from build123d import *

# Parameters (mm, degrees)
F1_DEPTH = 10
F2_R     = 10
F3_R     = 10


with BuildPart() as f1:
    # F0 (on Top) → F1 (new body)
    with BuildSketch(Plane.XY):
        with BuildLine():
            Line((-14.6, -8.429314), (-14.6, -20.293841))
            ThreePointArc((-14.6, -20.293841), (0, -25), (14.6, -20.293841))
            Line((14.6, -20.293841), (14.6, -8.429314))
            Line((14.6, -8.429314), (0, -16.858628))
            Line((0, -16.858628), (-14.6, -8.429314))
        make_face()
        with BuildLine():
            ThreePointArc((14.6, -20.293841), (22.248595, -11.401754), (25, 0))
            ThreePointArc((25, 0), (-11.401754, 22.248595), (-14.6, -20.293841))
            Line((-14.6, -20.293841), (-14.6, -8.429314))
            Line((-14.6, -8.429314), (-14.6, 8.429314))
            Line((-14.6, 8.429314), (0, 16.858628))
            Line((0, 16.858628), (14.6, 8.429314))
            Line((14.6, 8.429314), (14.6, -8.429314))
            Line((14.6, -8.429314), (14.6, -20.293841))
        make_face()
        with BuildLine():
            ThreePointArc((14.6, -20.293841), (0, -25), (-14.6, -20.293841))
            Line((-14.6, -20.293841), (-14.6, -104.361953))
            Line((-14.6, -104.361953), (14.6, -104.361953))
            Line((14.6, -104.361953), (14.6, -20.293841))
        make_face()
    extrude(amount=F1_DEPTH)

    # F2
    f2_edges = [f1.edges().sort_by_distance(p)[0] for p in [
        (14.6, -20.293841, 5),
    ]]
    fillet(f2_edges, radius=F2_R)

    # F3
    f3_edges = [f1.edges().sort_by_distance(p)[0] for p in [
        (-14.6, -20.293841, 5),
        (-14.6, -104.361953, 5),
        (14.6, -104.361953, 5),
    ]]
    fillet(f3_edges, radius=F3_R)


solid = f1.part
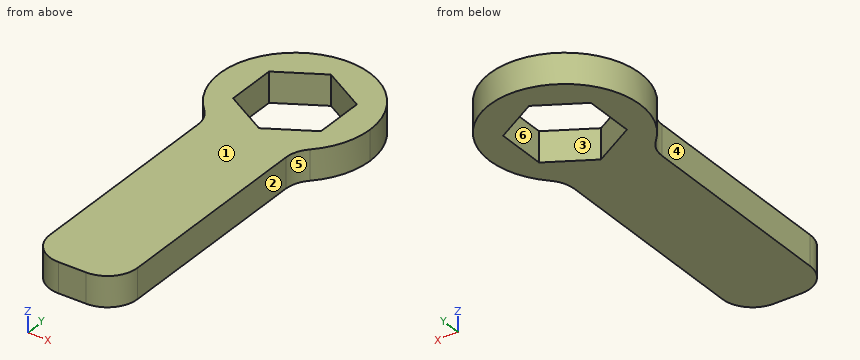
Input: part model. Units: mm. Frame: model coordinates. Face numbers are marked on the shaded views. A direction names the side the tool comes from. Give positions to 0.01 mm unless a question says otherwise; leave off trailing zeros. Order: outer loops, then holes, each group sorted by start corner. A loop starts at its lowest first (then second) coordinate and runs counter-clockwise, first axis right, second up. Notation, with made-up numbers: (67.5, 82.25) -> (89.5, 82.25) arc R27 ccw to (89.5, 109.25) -> close; hole circle Ø3 at (-10, 50.5). An arc over 180 degrees is marked (long way). Use one line per item in the form item = value.
1) Mould query, pull axis X, two halves, no side actions, for the marked faces 1, 2, 3 and 4. Classes: pulls with the +X half, pulls with the -X half, needs draft (parallel to the pull), parting line crosses it, or undercut.
Response values:
face_1 = needs draft
face_2 = pulls with the +X half
face_3 = undercut
face_4 = pulls with the -X half
2) Section C-C, the plane x = 1.5. Return loops of the section in (y, z), and give its area (3 significant figures).
Response values:
outline = (-104.36, 0) -> (-15.99, 0) -> (-15.99, 10) -> (-104.36, 10) -> close; (15.99, 0) -> (24.95, 0) -> (24.95, 10) -> (15.99, 10) -> close
area = 973 mm^2
3) Section A-A, the plane z = 3.75. Return loops of the section in (x, y).
Response values:
outline = (-17.57, -17.78) arc R10 cw to (-14.6, -24.9) -> (-14.6, -94.36) arc R10 ccw to (-4.6, -104.36) -> (4.6, -104.36) arc R10 ccw to (14.6, -94.36) -> (14.6, -24.9) arc R10 cw to (17.57, -17.78) arc R25 ccw to (25, 0) arc R25 ccw (long way) to start; hole (-14.6, -8.43) -> (0, -16.86) -> (14.6, -8.43) -> (14.6, 8.43) -> (0, 16.86) -> (-14.6, 8.43) -> close
4) Reachability of the marked faces 5 and 6 from +Z, -Z, +X, -X, +Y, -Y: full face, straight path, thin tool, end or side. Return the list, or none.
Response values:
face_5 = +Z, -Z, +X, -Y
face_6 = +Z, -Z
5) First-contact query: pin 1 Ø10 at (x, y) = (5, -18.5) entering from -Z; pin 2 Ø6 at (x, z) = (12.5, 7.5) entering from +Y; pin 3 Ø5 at (x, y) = (-18.5, -34.5) entering from +Z; pin 4 Ø5 at (x, z) = (9, 2.5) entering from -Y. Flat tips, straight axial feed; report the tip coordinate or a pass-through.
Response values:
pin_1 = 0
pin_2 = 23.12
pin_3 = through
pin_4 = -104.18
6) Section B-B, the plane x = -9. Return loops of the section in (y, z).
Response values:
outline = (-103.34, 0) -> (-11.66, 0) -> (-11.66, 10) -> (-103.34, 10) -> close; (11.66, 0) -> (23.32, 0) -> (23.32, 10) -> (11.66, 10) -> close
7) Section D-D, the plane y = -44. Return loops of the section in (x, z).
Response values:
outline = (-14.6, 0) -> (14.6, 0) -> (14.6, 10) -> (-14.6, 10) -> close
8) Line query: probe 1 along Y at (x, z) = (0, 9); probe 2 along X at (y, z) = (-75.5, 6.5); probe 3 along X at (y, z) = (14.5, 6.25). Output: solid intervals per line, ascending.
Response values:
probe_1 = -104.36 to -16.86, 16.86 to 25
probe_2 = -14.6 to 14.6
probe_3 = -20.37 to -4.09, 4.09 to 20.37
